```python
from build123d import *

# Parameters (mm, degrees)
ESQUISSE1_W             = 180
ESQUISSE1_H             = 90
BOSS_EXTRU_1_DEPTH      = 5
ESQUISSE2_W             = 180
ESQUISSE2_H             = 90
ESQUISSE2_W_2           = 170
ESQUISSE2_H_2           = 80
BOSS_EXTRU_2_DEPTH      = 30
ESQUISSE3_R             = 11.5
ESQUISSE3_R_2           = 6
ENL_V_MAT_EXTRU_1_DEPTH = 5
ESQUISSE4_W             = 12
ESQUISSE4_H             = 13
ENL_V_MAT_EXTRU_2_DEPTH = 5


with BuildPart() as part:
    # Esquisse1 → Boss.-Extru.1 (new body)
    with BuildSketch(Plane.XY):
        with Locations((90, 45)):
            Rectangle(ESQUISSE1_W, ESQUISSE1_H)
    extrude(amount=BOSS_EXTRU_1_DEPTH)

    # Esquisse2 → Boss.-Extru.2 (add)
    with BuildSketch(Plane.XY.offset(5)):
        with Locations((90, 45)):
            Rectangle(ESQUISSE2_W, ESQUISSE2_H)
        with Locations((90, 45)):
            Rectangle(ESQUISSE2_W_2, ESQUISSE2_H_2, mode=Mode.SUBTRACT)
    extrude(amount=BOSS_EXTRU_2_DEPTH)

    # Esquisse3 → Enlèv. mat.-Extru.1 (cut)
    with BuildSketch(Plane(origin=(0, 0, 0), x_dir=(-1, 0, 0), z_dir=(0, 0, -1))):
        with Locations((-140, 45)):
            Circle(ESQUISSE3_R)
        with Locations((-40, 56)):
            Circle(ESQUISSE3_R_2)
        with Locations((-40, 34)):
            Circle(ESQUISSE3_R_2)
        with Locations((-51, 45)):
            Circle(ESQUISSE3_R_2)
        with Locations((-29, 45)):
            Circle(ESQUISSE3_R_2)
    extrude(amount=-ENL_V_MAT_EXTRU_1_DEPTH, mode=Mode.SUBTRACT)

    # Esquisse4 → Enlèv. mat.-Extru.2 (cut)
    with BuildSketch(Plane.ZY):
        with Locations((27, 26.5)):
            Rectangle(ESQUISSE4_W, ESQUISSE4_H)
    extrude(amount=-ENL_V_MAT_EXTRU_2_DEPTH, mode=Mode.SUBTRACT)


solid = part.part
```
Verification items for the finished model (mm, model axes). A direction names the side the tool comes from. Round coordinates to 2 decimals unless told otherwise and drop trailing zeros. Order: outer loops, then holes, each group sorted by start corner. A loop starts at its lowest first (then second) coordinate and runs counter-clockwise, first axis right, second up. Notation, with made-up numbers: (88, -8) -> (98, -8) arc R29 ccw to (98, 13) -> close; hole circle Ø1 at (31.5, 52.5). An arc over 180 degrees is marked (long way). Put each result on its own line as item: value. Start each with the question number.
(1) Tool access check on faces 5 (the face through (2, 20, 27)), 6 (the face through (89, 85, 20)), 7 (the face through (35, 45, 2)). Record the directions out of +Z, -Z, +X, -X, +Y, -Y that give a thin tool (end or side, any length) a straight path to the whole face; none if there is none.
(2) Section check A-A (y = 23). Enter the section's corners in (x, z), then the cut area to 3 significant figures.
(3) Material ranges on line 1 along X through (y, z) = (42.5, 17.5); line 2 along Y through (x, z) = (24, 15); line 3 along Y through (x, z) = (29, 2), recorded low to high.
(4) Section check C-C (y = 45). Enter the section's corners in (x, z).
(5) Draft check along Z on faces 1 (the face through (5, 44, 20)), 2 (the face through (89.6, 85.2, 35)), 3 (the face through (2, 26, 21)), 4 (the face through (2, 26, 33)). Enter one of: +Z half, -Z half, draft (parallel to the pull), parting line (faces both ways), or undercut.
(6) Depth check by flat-ended pin: pin 1 Ø1 at (x, y) = (79.5, 75.5) entering from +Z; pin 2 Ø9.5 at (x, y) = (51, 45) entering from +Z. Enter the tip coordinate at first touch or a pass-through.
(7) Section check B-B (x = 51). Enter the section's corners in (y, z).
(8) Section check D-D (z = 11). Enter the section's corners in (x, y).
Completed:
1. face 5: -X
1. face 6: +Z
1. face 7: +Z, -Z
2. outline: (0, 0) -> (180, 0) -> (180, 35) -> (175, 35) -> (175, 5) -> (5, 5) -> (5, 21) -> (0, 21) -> close; (0, 33) -> (5, 33) -> (5, 35) -> (0, 35) -> close
2. area: 1,140 mm2
3. line 1: x = 0 to 5, 175 to 180
3. line 2: y = 0 to 5, 85 to 90
3. line 3: y = 0 to 39, 51 to 90
4. outline: (0, 0) -> (23, 0) -> (23, 5) -> (5, 5) -> (5, 35) -> (0, 35) -> close; (35, 0) -> (45, 0) -> (45, 5) -> (35, 5) -> close; (57, 0) -> (128.5, 0) -> (128.5, 5) -> (57, 5) -> close; (151.5, 0) -> (180, 0) -> (180, 35) -> (175, 35) -> (175, 5) -> (151.5, 5) -> close
5. face 1: draft
5. face 2: +Z half
5. face 3: undercut
5. face 4: undercut
6. pin 1: stops at z = 5
6. pin 2: passes through
7. outline: (0, 0) -> (39, 0) -> (39, 5) -> (5, 5) -> (5, 35) -> (0, 35) -> close; (51, 0) -> (90, 0) -> (90, 35) -> (85, 35) -> (85, 5) -> (51, 5) -> close
8. outline: (0, 0) -> (180, 0) -> (180, 90) -> (0, 90) -> close; hole (5, 5) -> (175, 5) -> (175, 85) -> (5, 85) -> close
